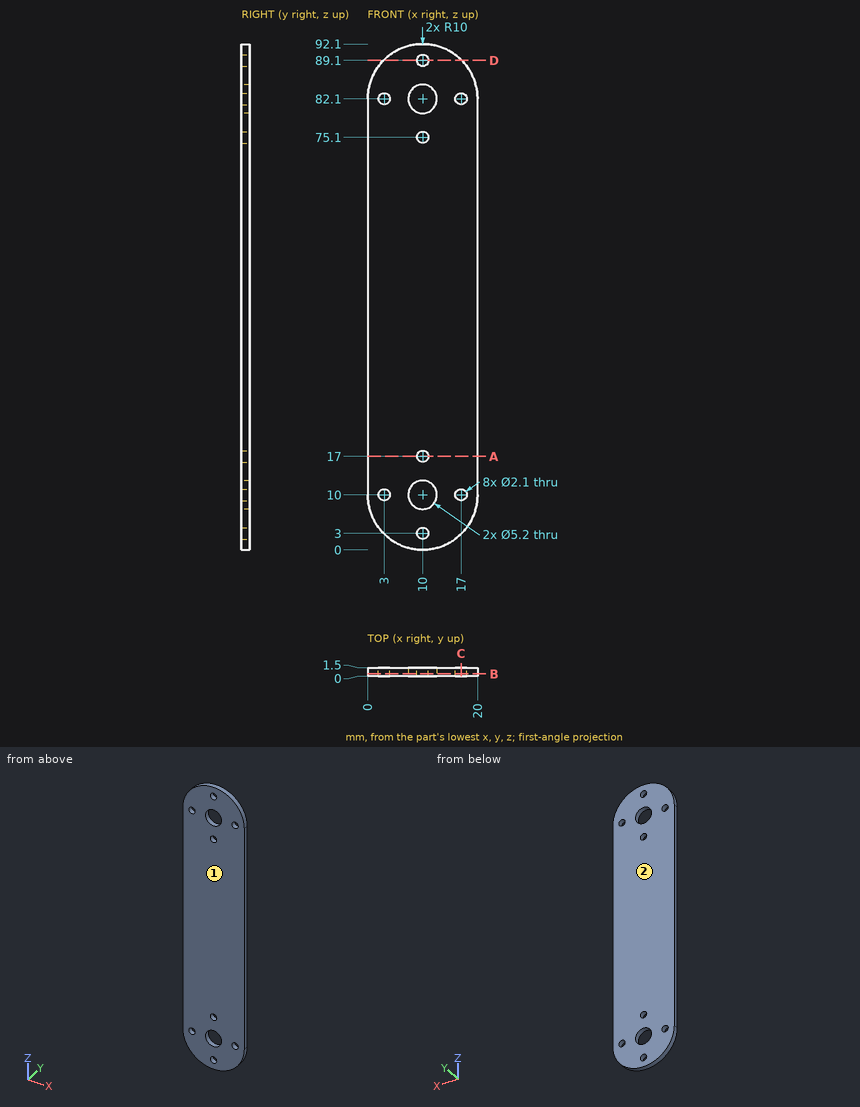
Print and shaded views of the part. All mm, measured from the part's lowest x, y and z. Round coordinates to 2 decimals unless told otherwise and drop trailing zeros. Order: outer loops, then holes, each group sorted by start corner. A loop starts at its lowest first (then second) coordinate and runs counter-clockwise, first axis right, second up.
Q1. Slice it at D-D (z = 89.1). Write the cut outline in (x, y), and give its area (3 significant figures).
Q2. Slice it at A-A (z = 17). Write the cut outline in (x, y), and give its area (4 significant figures).
Q3. Two-plate mould, pull along Y, no slides. Class the marked faces 1 and 2: pulls with the +Y half, pulls with the -Y half, needs draft (parallel to the pull), parting line crosses it, or undercut.
Q4. Slice it at B-B (y = 0.4). State how many separate pieces and enclosed holes the cut face has, and give its area (3 significant figures).
Q5. Slice it at C-C (x = 17). Write the cut outline in (y, z).
Q6. Drop a flat-ended pin along its axis: pin 1 (1.9 mm diameter, centred on x = 3, z = 10, fed in from +Y). Give the stop position or say it passes through.
Q7. Wall check: L1, parallel to X at y = 0.9, z = 10; L2, parallel to Z at x = 17.5, y = 0.5; L3, parallel to Z at x = 2.75, y = 1.2. Give the ranges that are in metal, low to high.
Results below:
1. outline: (2.86, 0) - (8.95, 0) - (8.95, 1.5) - (2.86, 1.5) - close; (11.05, 0) - (17.14, 0) - (17.14, 1.5) - (11.05, 1.5) - close
1. area: 18.3 mm2
2. outline: (0, 0) - (8.95, 0) - (8.95, 1.5) - (0, 1.5) - close; (11.05, 0) - (20, 0) - (20, 1.5) - (11.05, 1.5) - close
2. area: 26.85 mm2
3. face 1: pulls with the -Y half
3. face 2: pulls with the +Y half
4. separate pieces: 1
4. enclosed holes: 10
4. area: 1,690 mm2
5. outline: (0, 2.86) - (1.5, 2.86) - (1.5, 8.95) - (0, 8.95) - close; (0, 11.05) - (1.5, 11.05) - (1.5, 81.05) - (0, 81.05) - close; (0, 83.15) - (1.5, 83.15) - (1.5, 89.24) - (0, 89.24) - close
6. pin 1: passes through
7. L1: x = 0 to 1.95, 4.05 to 7.4, 12.6 to 15.95, 18.05 to 20
7. L2: z = 3.39 to 9.08, 10.92 to 81.18, 83.02 to 88.71
7. L3: z = 3.11 to 8.98, 11.02 to 81.08, 83.12 to 88.99
